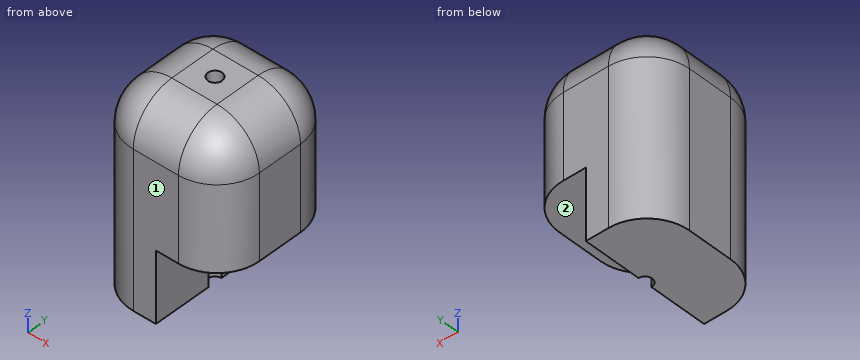
```python
from build123d import *

# Parameters (mm, degrees)
SKETCH_W        = 9.2
SKETCH_H        = 9.2
PAD_DEPTH       = 14
SKETCH001_R     = 0.5
POCKET_DEPTH    = 14.001
FILLET_R        = 3
SKETCH002_W     = 5.20137
SKETCH002_H     = 9.517286
POCKET001_DEPTH = 5


with BuildPart() as part:
    # Sketch → Pad (new body)
    with BuildSketch(Plane.XY):
        Rectangle(SKETCH_W, SKETCH_H)
    extrude(amount=PAD_DEPTH)

    # Sketch001 (on Face6 of Pad) → Pocket (cut, through all)
    with BuildSketch(Plane.XY.offset(14)):
        Circle(SKETCH001_R)
    extrude(amount=-POCKET_DEPTH, mode=Mode.SUBTRACT)

    # Fillet
    fillet_edges = [part.edges().sort_by_distance(p)[0] for p in [
        (0, 4.6, 14),
        (4.6, 4.6, 7),
        (4.6, 0, 14),
        (-4.6, 4.6, 7),
        (-4.6, 0, 14),
        (4.6, -4.6, 7),
        (-4.6, -4.6, 7),
        (0, -4.6, 14),
    ]]
    fillet(fillet_edges, radius=FILLET_R)

    # Sketch002 (on Face2 of Fillet) → Pocket001 (cut)
    with BuildSketch(Plane(origin=(0, 0, 0), x_dir=(1, 0, 0), z_dir=(0, 0, -1))):
        with Locations((2.600685, 0.034579)):
            Rectangle(SKETCH002_W, SKETCH002_H)
    extrude(amount=-POCKET001_DEPTH, mode=Mode.SUBTRACT)


solid = part.part
```
Geometry: final body of the model. Coordinates: model frame, mm. Face numbers are marked on the shaded views. A direction names the side the tool comes from. Give positions to 0.01 mm unless a question says otherwise; leave off trailing zeros. Write each loop counter-clockwise with the first axis right and the second up, starting at its lowest first coordinate (ties: lowest second). Pieces come first, ordered by that corner, then holes.
1. Section query C-C, the plane x = 0.25. Return loops of the section in (y, z).
2. Section query A-A, the plane y = 0. Return loops of the section in (x, z).
3. Line query: probe 1 along X at (y, z) = (0, 8); probe 2 along X at (y, z) = (-0.75, 1.75). Output: solid intervals per line, ascending.
4. Section query B-B, the plane z = 5.5. Return loops of the section in (x, y).
5. Reachability of the marked faces 1 and 2 from +Z, -Z, +X, -X, +Y, -Y: full face, straight path, thin tool, end or side. Return the list, or none.
6. Pin query (flat end, axial travel): P1, Ø1.5, axis at x = 2.5, y = 0.5, coming from the +Z side; P2, Ø1.4, axis at x = 1.5, y = 2, coming from the -Z side; P3, Ø1, axis at x = -2.5, z = 9.5, coming from the +Y side. Return the tip coordinate at first contact, or that it passes through.
7. Section query D-D, the plane y = 2.5. Return loops of the section in (x, z).
Computed:
1. outline: (-4.6, 5) - (-0.43, 5) - (-0.43, 14) - (-1.6, 14) arc R3 ccw to (-4.6, 11) - close; (0.43, 5) - (4.6, 5) - (4.6, 11) arc R3 ccw to (1.6, 14) - (0.43, 14) - close
2. outline: (-4.6, 0) - (-0.5, 0) - (-0.5, 14) - (-1.6, 14) arc R3 ccw to (-4.6, 11) - close; (0.5, 5) - (4.6, 5) - (4.6, 11) arc R3 ccw to (1.6, 14) - (0.5, 14) - close
3. probe 1: x = -4.6 to -0.5, 0.5 to 4.6
3. probe 2: x = -4.6 to 0
4. outline: (-4.6, -1.6) arc R3 ccw to (-1.6, -4.6) - (1.6, -4.6) arc R3 ccw to (4.6, -1.6) - (4.6, 1.6) arc R3 ccw to (1.6, 4.6) - (-1.6, 4.6) arc R3 ccw to (-4.6, 1.6) - close; hole circle Ø1 at (0, 0)
5. face 1: +Z, -Z, +X, -X, -Y
5. face 2: -Z, +X, +Y, -Y
6. P1: stops at z = 14
6. P2: stops at z = 5
6. P3: stops at y = 4.57
7. outline: (-4.46, 0) - (0, 0) - (0, 5) - (4.46, 5) - (4.46, 11) arc R2.86 ccw to (1.6, 13.86) - (-1.6, 13.86) arc R2.86 ccw to (-4.46, 11) - close
